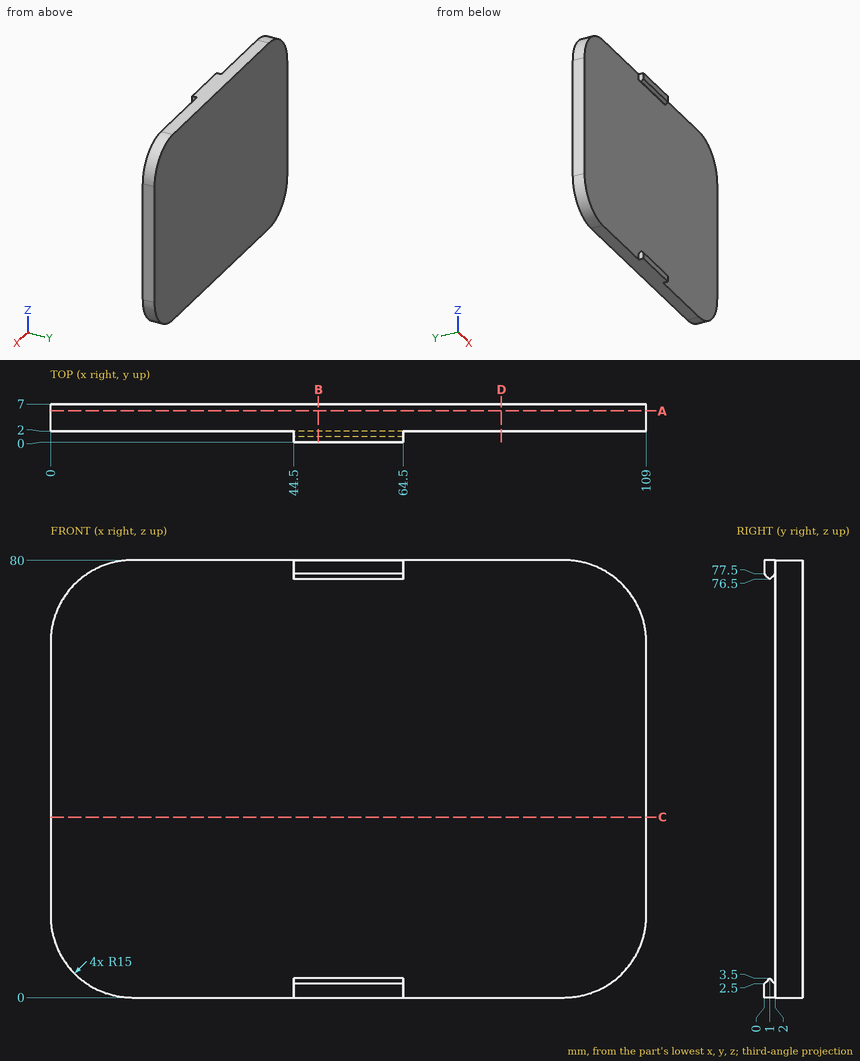
Check sheet for the drawn part. Datum: minimum x, y, z corner. Units: mm. Coordinates: 2 decimals unless noted, no trailing zeros. Loops run counter-clockwise (first coordinate to the right, second up) from the corner with the lowest first, then second, coordinate; pieces in that order, holes last. Notation, with made-up numbers: (-11.75, 51) -> (15.25, 51) arc R30 cw to (15.25, 83) -> close; hole circle Ø10 at (-23.75, -15.5). An arc over 180 degrees is marked (long way). Answer in a Markdown table with one row per item.
1. Sectioned sample at A-A, the plane y = 5.75. Record the boundary of the cut face in (x, z), then the cut area to 3 significant figures.
Check values:
| item | result |
|---|---|
| outline | (0, 15) arc R15 ccw to (15, 0) -> (94, 0) arc R15 ccw to (109, 15) -> (109, 65) arc R15 ccw to (94, 80) -> (15, 80) arc R15 ccw to (0, 65) -> close |
| area | 8,530 mm2 |
2. Sectioned sample at B-B, the plane x = 49. Record the boundary of the cut face in (y, z), then the cut area to 3 significant figures.
Check values:
| item | result |
|---|---|
| outline | (0, 0) -> (7, 0) -> (7, 80) -> (0, 80) -> (0, 77.5) -> (1, 76.5) -> (2, 77.5) -> (2, 2.5) -> (1, 3.5) -> (0, 2.5) -> close |
| area | 412 mm2 |
3. Sectioned sample at C-C, the plane z = 33. Record the boundary of the cut face in (x, y).
Check values:
| item | result |
|---|---|
| outline | (0, 2) -> (109, 2) -> (109, 7) -> (0, 7) -> close |
4. Material ranges on line 1 along Y through (x, z) = (102, 34.5); line 2 along X through (y, z) = (4.25, 68); line 3 along X through (y, z) = (2.25, 69), recorded low to high. Write a range as [from, to].
Check values:
| item | result |
|---|---|
| line 1 | y = [2, 7] |
| line 2 | x = [0.3, 108.7] |
| line 3 | x = [0.54, 108.46] |
5. Sectioned sample at D-D, the plane x = 82.5. Record the boundary of the cut face in (y, z).
Check values:
| item | result |
|---|---|
| outline | (2, 0) -> (7, 0) -> (7, 80) -> (2, 80) -> close |
6. Go/stop test with flat-tipped pins: pin 1 (2 mm diameter, centred on y = 1.5, z = 77.5, fed in from +X); pin 2 (2 mm diameter, centred on x = 69, z = 68, fed in from -Y); pin 3 (1 mm diameter, centred on x = 36, y = 4, fed in from -Z); pin 4 (1.6 mm diameter, centred on y = 1, z = 78.5, fed in from -X). Record where each tip stops, or that it passes through.
Check values:
| item | result |
|---|---|
| pin 1 | stops at x = 103.47 |
| pin 2 | stops at y = 2 |
| pin 3 | stops at z = 0 |
| pin 4 | stops at x = 44.5 |
